Design review of the part built by this model. Coordinates are the model's own, in mm. A direction names the side the tool comes from. Coordinates: 2 decimals unless noted, no trailing zeros. Order: outer loops, then holes, each group sorted by start corner. A loop starts at its lowest first (then second) coordinate and runs counter-clockwise, first axis right, second up. Notation, with made-up numbers: M -33,40 L -18,40 A27 ccw -18,79 Z; hole C -25.75,20.5 d2. An arc over 180 degrees is marked long. Answer as a JSON object with one key per item and string values.
from build123d import *

# Parameters (mm, degrees)
SKETCH_1_W          = 150
SKETCH_1_H          = 93
EXTRUDE_2_DEPTH     = 2
SKETCH_2_W          = 130
SKETCH_2_H          = 83
EXTRUDE_3_DEPTH     = 25
SKETCH_3_W          = 126
SKETCH_3_H          = 79
CUT_EXTRUDE_1_DEPTH = 2
SKETCH_4_W          = 126
SKETCH_4_H          = 79
CUT_EXTRUDE_2_DEPTH = 20


with BuildPart() as part:
    # 草图1 → 凸台-拉伸2 (new body)
    with BuildSketch(Plane.XY):
        with Locations((8.786617008, -6.973744962)):
            Rectangle(SKETCH_1_W, SKETCH_1_H)
    extrude(amount=EXTRUDE_2_DEPTH)

    # 草图2 → 凸台-拉伸3 (add)
    with BuildSketch(Plane.XY.offset(2)):
        with Locations((8.786617008, -6.973744962)):
            Rectangle(SKETCH_2_W, SKETCH_2_H)
    extrude(amount=EXTRUDE_3_DEPTH)

    # 草图3 → 切除-拉伸1 (cut)
    with BuildSketch(Plane(origin=(0, 0, 0), x_dir=(-1, 0, 0), z_dir=(0, 0, -1))):
        with Locations((-8.786617008, -6.973744962)):
            Rectangle(SKETCH_3_W, SKETCH_3_H)
    extrude(amount=-CUT_EXTRUDE_1_DEPTH, mode=Mode.SUBTRACT)

    # 草图4 → 切除-拉伸2 (cut)
    with BuildSketch(Plane.XY.offset(27)):
        with Locations((8.786617008, -6.973744962)):
            Rectangle(SKETCH_4_W, SKETCH_4_H)
    extrude(amount=-CUT_EXTRUDE_2_DEPTH, mode=Mode.SUBTRACT)


solid = part.part
1) Tool access review of faces 1 (the flat face through (8, -6, 7)), 2 (the flat face through (8, -48.474, 14)), 3 (the flat face through (8, 34.526, 14)), 4 (the flat face through (10, -6, 2)): name each direction out of +Z, -Z, +X, -X, +Y, -Y from which nothing blocks a thin tool from reaching the whole face with its end or side.
Taken from the geometry:
{"face 1": "+Z", "face 2": "+Z, +X, -X, -Y", "face 3": "+Z, +X, -X, +Y", "face 4": "-Z"}
2) To check wall thickness, follow L1, parallel to Y at x = 25, z = 16; L2, parallel to X at y = -45, z = 20.5; L3, parallel to Z at x = 48, y = -40. State the ranges of each line that lie inside material, in increasing order.
Taken from the geometry:
{"L1": "y = -48.47 to -46.47, 32.53 to 34.53", "L2": "x = -56.21 to -54.21, 71.79 to 73.79", "L3": "z = 2 to 7"}
3) Mouldability with a two-part tool opening along X and no side actions: class faces 5 (the flat face through (8, -48, 0)), 6 (the flat face through (-56.213, -8, 14)), 7 (the flat face through (73.787, -8, 14)), 8 (the flat face through (-54.213, -8, 17)) as released by +X, released by -X, zero draft, split by the parting line, or undercut.
Taken from the geometry:
{"face 5": "zero draft", "face 6": "released by -X", "face 7": "released by +X", "face 8": "undercut"}
4) Add section D-D (z = 4.25). State the section outline as (x, y) points.
Taken from the geometry:
{"outline": "M -56.21,-48.47 L 73.79,-48.47 L 73.79,34.53 L -56.21,34.53 Z"}
5) Insertion check: pin 1 Ø10 at (x, y) = (26, -12) entering from -Z; pin 2 Ø2 at (y, z) = (6, 7.5) entering from +X; pin 3 Ø12 at (x, z) = (-17, 14.5) entering from -Y. Each pin has a flat end and moves straight along its axis. Give the tip position at first contact, or say it passes through.
Taken from the geometry:
{"pin 1": "stops at z = 2", "pin 2": "stops at x = 73.79", "pin 3": "stops at y = -48.47"}
6) Add section A-A (x = -45.5). State the section outline as (y, z) points.
Taken from the geometry:
{"outline": "M -53.47,0 L -46.47,0 L -46.47,2 L 32.53,2 L 32.53,0 L 39.53,0 L 39.53,2 L 34.53,2 L 34.53,27 L 32.53,27 L 32.53,7 L -46.47,7 L -46.47,27 L -48.47,27 L -48.47,2 L -53.47,2 Z"}
7) Add section C-C (y = -11). State the section outline as (x, z) points, and give its area (3 significant figures).
Taken from the geometry:
{"outline": "M -66.21,0 L -54.21,0 L -54.21,2 L 71.79,2 L 71.79,0 L 83.79,0 L 83.79,2 L 73.79,2 L 73.79,27 L 71.79,27 L 71.79,7 L -54.21,7 L -54.21,27 L -56.21,27 L -56.21,2 L -66.21,2 Z", "area": "778 mm2"}
8) Add section B-B (z = 11). State the section outline as (x, y) points, and give its area (3 significant figures).
Taken from the geometry:
{"outline": "M -56.21,-48.47 L 73.79,-48.47 L 73.79,34.53 L -56.21,34.53 Z; hole M -54.21,-46.47 L 71.79,-46.47 L 71.79,32.53 L -54.21,32.53 Z", "area": "836 mm2"}
